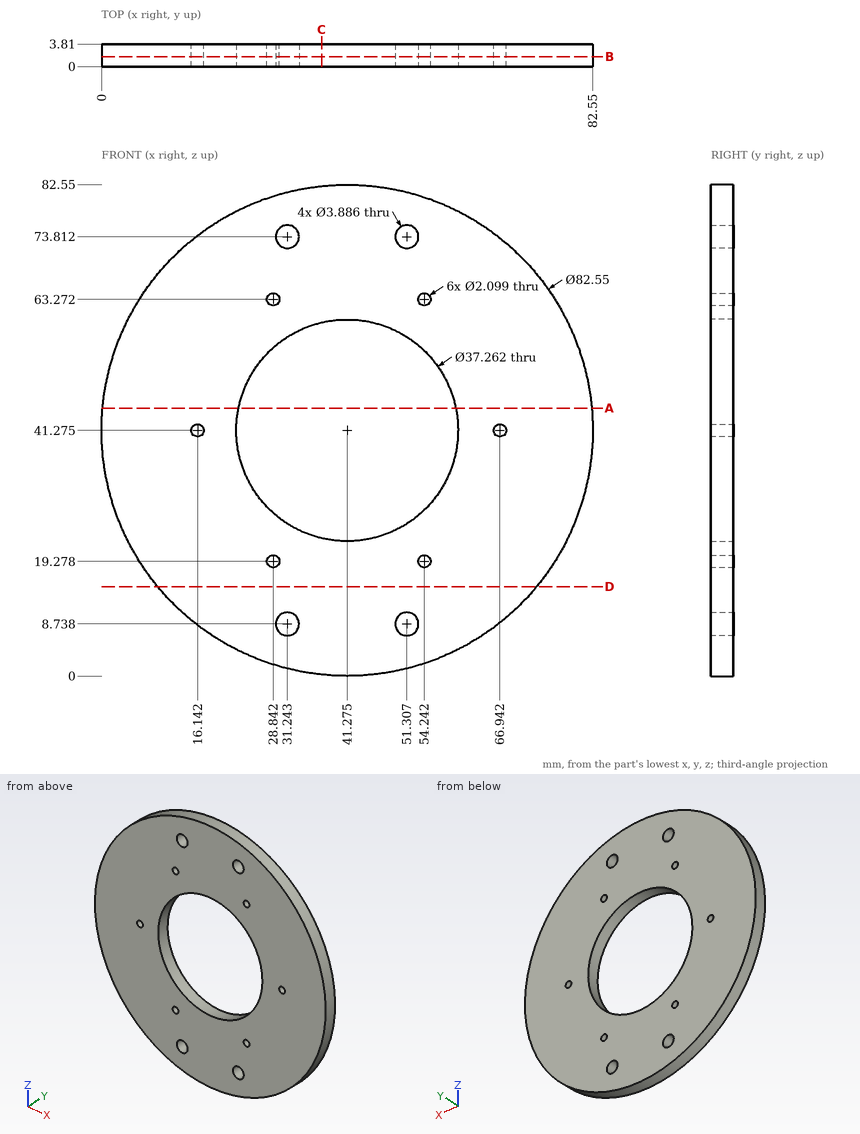
Verification items for this drawing (mm, ordinates from the low corner). Coordinates: 2 decimals unless noted, no trailing zeros. Loops run counter-clockwise (first coordinate to the right, second up) from the corner with the lowest first, then second, coordinate; pieces in that order, holes last. Notation, with made-up numbers: (24.25, 65.25) -> (79.25, 65.25) arc R31 cw to (79.25, 97.25) -> close; hole circle Ø4 at (-36.75, -20.75). An arc over 180 degrees is marked (long way). Put each result on its own line as item: value.
1. Section check D-D, the plane z = 15. Record the boundary of the cut face in (x, y).
Result set:
outline: (9.44, 0) -> (73.11, 0) -> (73.11, 3.81) -> (9.44, 3.81) -> close
2. Section check C-C, the plane x = 37. Record the boundary of the cut face in (y, z).
Result set:
outline: (0, 0.22) -> (3.81, 0.22) -> (3.81, 23.14) -> (0, 23.14) -> close; (0, 59.41) -> (3.81, 59.41) -> (3.81, 82.33) -> (0, 82.33) -> close
3. Section check B-B, the plane y = 1.7. Give the number of separate pieces and of enclosed holes in the cut face, then the cut area to 3 significant figures.
Result set:
separate pieces: 1
enclosed holes: 11
area: 4,190 mm^2
4. Thickness scan on line 1 (X direction, y = 3.5, z = 10.5) (1 decimal); line 2 (Z direction, x = 38.5, y = 0.5); line 3 (Z direction, x = 48, y = 3.3). Record the ranges inside material, lowest first.
Result set:
line 1: x = 13.8 to 30.4, 32.1 to 50.5, 52.1 to 68.8
line 2: z = 0.09 to 22.85, 59.7 to 82.46
line 3: z = 0.55 to 23.9, 58.65 to 82
5. Gauge pin test, flat ends, axial feed: P1, Ø2, axis at y = 0.5, z = 72.5, coming from the -X side (1 decimal); P2, Ø1, axis at x = 12.5, y = 1, coming from the -Z side (1 decimal); P3, Ø1.5, axis at x = 17.5, y = 3, coming from the -Z side. Record the tip position at first contact, or that the pin passes through.
Result set:
P1: stops at x = 13.2
P2: stops at z = 11.2
P3: stops at z = 7.02
6. Section check A-A, the plane z = 45. Record the boundary of the cut face in (x, y).
Result set:
outline: (0.17, 0) -> (23.02, 0) -> (23.02, 3.81) -> (0.17, 3.81) -> close; (59.53, 0) -> (82.38, 0) -> (82.38, 3.81) -> (59.53, 3.81) -> close
